Design review of the part shown in the three views and the two pictorial views. Dimensions are in mm from the part's minimum x, y and z. A direction names the side the tool comes from. Coordinates: 2 decimals unless noted, no trailing zeros. Write each loop counter-clockwise with the first axis right and the second up, starting at its lowest first coordinate (ties: lowest second). Pieces come first, ordered by that corner, then holes. Notation, with made-up numbers: (-17, -17) -> (-12, -17) arc R8 cw to (-12, -6) -> close; hole circle Ø2 at (-11.5, 50). An arc over 180 degrees is marked (long way). Write each question's results on one line, items separated by ' | '.
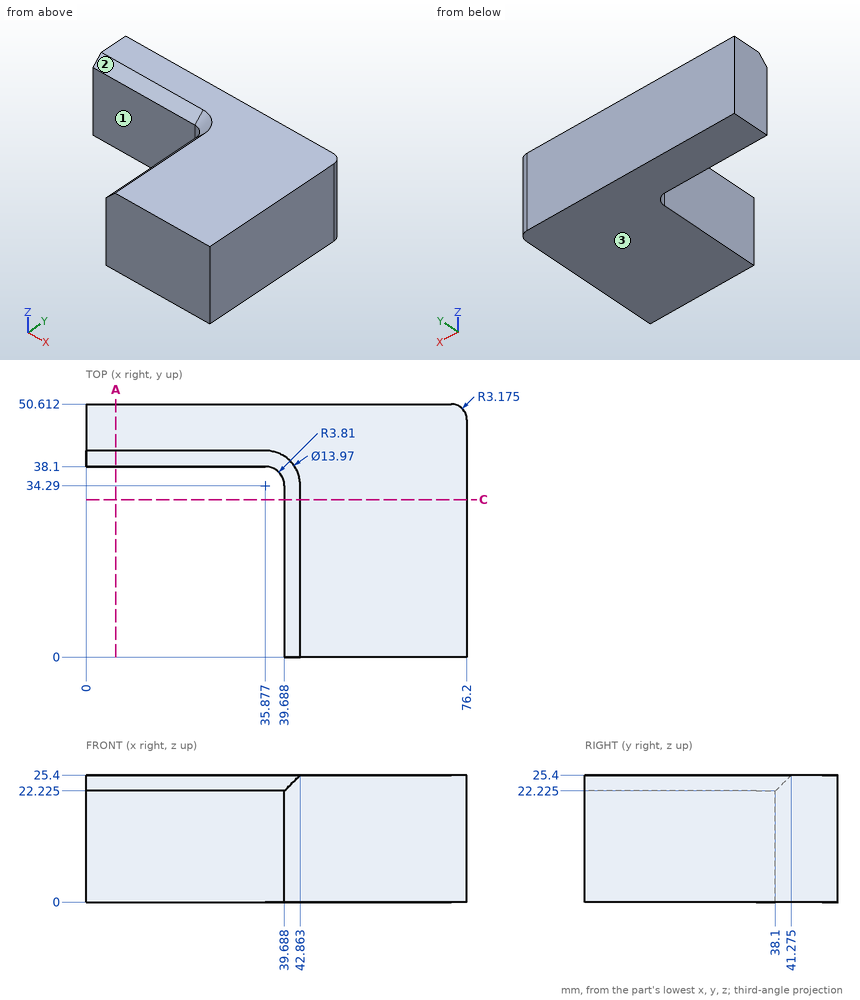
Q1. Add section A-A (x = 6). Write out the cut boundary in (y, z) (1 decimal).
Solution:
outline: (38.1, 0) -> (50.6, 0) -> (50.6, 25.4) -> (41.3, 25.4) -> (38.1, 22.2) -> close
Q2. Machinability: for the marked faces 1, 2 and 3, which of the approach directions +Z, -Z, +X, -X, +Y, -Y give a long, thin tool a straight path to every point of the face, cutting with its end or side? Answer none if there is none.
Solution:
face 1: +Z, -Z, -X, -Y | face 2: +Z, -X, -Y | face 3: -Z, +X, -X, +Y, -Y
Q3. Clearance check with flat-ended pins moving along their axes: P1, Ø3, axis at y = 25, z = 20, coming from the -X side; P2, Ø5, axis at x = 59.5, y = 23.5, coming from the -Z side; P3, Ø2, axis at x = 10, z = 5.5, coming from the -Y side. State where each tip first meets the part, or that it passes through.
Solution:
P1: x = 39.69 | P2: z = 0 | P3: y = 38.1
Q4. Add section C-C (y = 31.5). Write out the cut boundary in (x, z) (1 decimal).
Solution:
outline: (39.7, 0) -> (76.2, 0) -> (76.2, 25.4) -> (42.9, 25.4) -> (39.7, 22.2) -> close
Q5. For line 1 (X direction, y = 22, z = 4); line 2 (Y direction, x = 6.5, z = 17.5); line 3 (Y direction, x = 11, z = 23.5) (1 decimal), list the stretches that pass through material, from the lowest coordinate up. Write a range as from..to.
Solution:
line 1: 39.69..76.2 | line 2: 38.1..50.61 | line 3: 39.4..50.6
